```python
from build123d import *

# Parameters (mm, degrees)
SKETCH1_R                     = 32.75
OUTER_DISK_DEPTH              = 2
ENCLOSEMENT_T                 = 2
HOOK_RELEASE_DEPTH            = 50.184601249
CIRPATTERN1_COUNT             = 2
CIRPATTERN1_ANGLE             = 90
SERVO_MOTOR_CUTOUT_DEPTH      = 50.184601249
SERVO_MOTOR_CUTOUT_DEPTH_BACK = 50.184601249
SKETCH3_R                     = 3
SKETCH3_R_2                   = 5.9
FILLET1_R                     = 1


with BuildPart() as part:
    # Sketch1 → Outer DIsk (new body)
    with BuildSketch(Plane(origin=(0, 0, 0), x_dir=(1, 0, 0), z_dir=(0, 1, 0))):
        with Locations(Location((0, 0, 0), (0, 0, 270))):
            Circle(SKETCH1_R)
    extrude(amount=OUTER_DISK_DEPTH)

    # Enclosement
    enclosement_openings = [part.faces().sort_by_distance(p)[0] for p in [
        (0, 2, 0),
    ]]
    offset(amount=ENCLOSEMENT_T, openings=enclosement_openings, kind=Kind.INTERSECTION)

    # Sketch2 → Hook Release (cut, symmetric)
    with BuildSketch(Plane(origin=(0, 0, 0), x_dir=(1, 0, 0), z_dir=(0, 1, 0))):
        Polygon((-2, 34.75), (-2, 28.75), (8, 28.75), (8, 30.75), (2, 30.75), (2, 34.75), align=None)
    hook_release = extrude(amount=HOOK_RELEASE_DEPTH, both=True, mode=Mode.SUBTRACT)

    # CirPattern1: Hook Release ×2 about axis
    cirpattern1_axis = Axis((0, 0, 0), (0, 1, 0))
    for i in range(1, CIRPATTERN1_COUNT):
        add(hook_release.rotate(cirpattern1_axis, i * CIRPATTERN1_ANGLE / (CIRPATTERN1_COUNT - 1)), mode=Mode.SUBTRACT)

    # Sketch3 → Servo Motor Cutout (cut, two sides: drawn at the far end of the back side and taken through both)
    with BuildSketch(Plane(origin=(0, 0, 0), x_dir=(1, 0, 0), z_dir=(0, 1, 0)).offset(-SERVO_MOTOR_CUTOUT_DEPTH_BACK)):
        with Locations((5.9, 0)):
            Circle(SKETCH3_R)
        Circle(SKETCH3_R_2)
    extrude(amount=SERVO_MOTOR_CUTOUT_DEPTH + SERVO_MOTOR_CUTOUT_DEPTH_BACK, mode=Mode.SUBTRACT)

    # Fillet1
    fillet1_edges = [part.edges().sort_by_distance(p)[0] for p in [
        (-28.75, -1, 2),
        (-28.75, -1, -8),
        (-30.75, -1, -8),
        (-30.75, -1, -2),
        (8, -1, -28.75),
        (-2, -1, -28.75),
        (8, -1, -30.75),
        (2, -1, -30.75),
    ]]
    fillet(fillet1_edges, radius=FILLET1_R - 0.0001)  # a hair under: the kernel refuses the full size


solid = part.part
```
Input: part model. Units: mm. Frame: model coordinates. A direction names the side the tool comes from. Coordinates: 2 decimals unless noted, no trailing zeros. Write each loop counter-clockwise with the first axis right and the second up, starting at its lowest first coordinate (ties: lowest second). Pieces come first, ordered by that corner, then holes. Notation, with made-up numbers: (54, 71) - (93, 71) arc R13 ccw to (93, 79) - close; hole circle Ø11 at (16.5, 88). An arc over 180 degrees is marked (long way). Put each result on its own line as item: value. Start each with the question number.
1) Reachability of faces 1 (the face through (-33, 0, 2)), 2 (the face through (-7, 0, 0)), 3 (the face through (3, -1, -28.75)), 4 (the face through (-2, 0, -33)) from +Z, -Z, +X, -X, +Y, -Y: full face, straight path, thin tool, end or side. Return the list, or none.
2) Mould query, pull axis X, two halves, no side actions, for faces 5 (the face through (23.77, -0.03, 25.35)), 6 (the face through (2, 0, -34)), 7 (the face through (-34, 0, -2)). Classes: pulls with the +X half, pulls with the -X half, needs draft (parallel to the pull), parting line crosses it, or undercut.
3) Cut plane D-D (x = -23.5). Return the cut outline in (y, z), plus the area to 3 significant figures.
4) Cut plane C-C (y = 0.75). Return the cut outline in (x, z), plus the area to 3 significant figures.
5) Cut plane B-B (x = 0). Return the cut outline in (y, z), plus the area to 3 significant figures.
6) Ray query, L1, parallel to X at y = -1.3, z = 0; L2, parallel to Z at x = 5.9, y = -0.5; L3, parallel to X at y = 1.5, z = 0. Return the intervals inside material, ascending.
7) Cut plane A-A (z = 0). Return the cut outline in (x, y), plus the area to 3 significant figures.
8) Contact query for flat-ended pins moving along their axis: pin 1 (1.6 mm diameter, centred on y = -1, z = -4.5, fed in from +X); pin 2 (2 mm diameter, centred on x = 6, y = -1, fed in from +Z); pin 3 (1 mm diameter, centred on y = -1, z = -3, fed in from -X). Output: stop coordinate, or through.
Resolved:
1. face 1: -X, +Y, -Y
1. face 2: +Y
1. face 3: +Y, -Y
1. face 4: -Z, +Y, -Y
2. face 5: parting line crosses it
2. face 6: undercut
2. face 7: needs draft
3. outline: (-2, -25.6) - (2, -25.6) - (2, -22.81) - (0, -22.81) - (0, 22.81) - (2, 22.81) - (2, 25.6) - (-2, 25.6) - close
3. area: 114 mm2
4. outline: (-34.69, -2) arc R34.75 ccw to (-2, -34.69) - (-2, -32.69) arc R32.75 cw to (-32.69, -2) - close; (-34.69, 2) - (-32.69, 2) arc R32.75 cw (long way) to (2, -32.69) - (2, -34.69) arc R34.75 ccw (long way) to start
4. area: 408 mm2
5. outline: (-2, -28.75) - (0, -28.75) - (0, -5.9) - (-2, -5.9) - close; (-2, 5.9) - (0, 5.9) - (0, 32.75) - (2, 32.75) - (2, 34.75) - (-2, 34.75) - close
5. area: 107 mm2
6. L1: x = -28.75 to -5.9, 8.9 to 34.75
6. L2: z = -34.25 to -30.75, -28.75 to -3, 3 to 34.25
6. L3: x = 32.75 to 34.75
7. outline: (-28.75, -2) - (-5.9, -2) - (-5.9, 0) - (-28.75, 0) - close; (8.9, -2) - (34.75, -2) - (34.75, 2) - (32.75, 2) - (32.75, 0) - (8.9, 0) - close
7. area: 101 mm2
8. pin 1: stops at x = 34.55
8. pin 2: stops at z = 34.39
8. pin 3: stops at x = -34.66
